```python
from build123d import *

# Parameters (mm, degrees)
SKETCH_1_R               = 3.5
SKETCH_1_R_2             = 2.5
EXTRUDE_1_DEPTH          = 3
CHAMFER_1_SIZE           = 0.1
CUT_EXTRUDE_2_DEPTH      = 6.787918451
CUT_EXTRUDE_2_DEPTH_BACK = 6.787918451
SKETCH_2_W               = 1
SKETCH_2_H               = 3.5


with BuildPart() as part:
    # 草图1 → 拉伸-薄壁1 (new body)
    with BuildSketch(Plane.XY):
        Circle(SKETCH_1_R)
        Circle(SKETCH_1_R_2, mode=Mode.SUBTRACT)
    extrude(amount=EXTRUDE_1_DEPTH)

    # 倒角1
    chamfer_1_edges = [part.edges().sort_by_distance(p)[0] for p in [
        (-3.5, 0, 0),
        (-2.5, 0, 0),
        (-3.5, 0, 3),
        (-2.5, 0, 3),
    ]]
    chamfer(chamfer_1_edges, length=CHAMFER_1_SIZE)

    # 草图2 → 切除-拉伸-薄壁2 (cut, two sides: drawn at the far end of the back side and taken through both)
    with BuildSketch(Plane(origin=(0, 0, 0), x_dir=(-1, 0, 0), z_dir=(0, 0, -1)).offset(-CUT_EXTRUDE_2_DEPTH_BACK)):
        with Locations((0, 1.75)):
            Rectangle(SKETCH_2_W, SKETCH_2_H)
    extrude(amount=CUT_EXTRUDE_2_DEPTH + CUT_EXTRUDE_2_DEPTH_BACK, mode=Mode.SUBTRACT)


solid = part.part
```
Build history of the part. All positions in model axes, mm. A direction names the side the tool comes from. Round coordinates to 2 decimals unless told otherwise and drop trailing zeros. Order: outer loops, then holes, each group sorted by start corner. A loop starts at its lowest first (then second) coordinate and runs counter-clockwise, first axis right, second up. Notation, with made-up numbers: (-39, -22.5) -> (-27, -22.5) arc R19 cw to (-27, -18.5) -> close; hole circle Ø9 at (0.25, -21). An arc over 180 degrees is marked (long way). Answer in a Markdown table with one row per item.
1) Band-saw the part on A-A on y = 0. Give the cut face in (x, z), and give its area (3 significant figures).
Values:
| item | result |
|---|---|
| outline | (-3.5, 0.1) -> (-3.4, 0) -> (-2.6, 0) -> (-2.5, 0.1) -> (-2.5, 2.9) -> (-2.6, 3) -> (-3.4, 3) -> (-3.5, 2.9) -> close; (2.5, 0.1) -> (2.6, 0) -> (3.4, 0) -> (3.5, 0.1) -> (3.5, 2.9) -> (3.4, 3) -> (2.6, 3) -> (2.5, 2.9) -> close |
| area | 5.96 mm2 |
2) Band-saw the part on B-B on x = 0. Give the cut face in (y, z).
Values:
| item | result |
|---|---|
| outline | (-3.5, 0.1) -> (-3.4, 0) -> (-2.6, 0) -> (-2.5, 0.1) -> (-2.5, 2.9) -> (-2.6, 3) -> (-3.4, 3) -> (-3.5, 2.9) -> close |
3) Wall check: L1, parallel to X at y = 0, z = 1.9; L2, parallel to Y at x = 0, z = 2.15; L3, parallel to X at y = 3, z = 1. Give the ranges that are in metal, low to high.
Values:
| item | result |
|---|---|
| L1 | -3.5 to -2.5, 2.5 to 3.5 |
| L2 | -3.5 to -2.5 |
| L3 | -1.8 to -0.5, 0.5 to 1.8 |
4) Which spindle directions (+Z, -Z, +X, -X, +Y, -Y) get a long thin tool onto all of the face, cutting with end or side? Do faces 4 (the flat face through (0.5, 3, 2)), 5 (the flat face through (1, -3, 3)). Say none if no direction does.
Values:
| item | result |
|---|---|
| face 4 | +Z, -Z, +Y |
| face 5 | +Z, +X, -X, +Y, -Y |
5) Band-saw the part on C-C on z = 1.8. Give the cut face in (x, y), and give its area (3 significant figures).
Values:
| item | result |
|---|---|
| outline | (-0.5, 2.45) -> (-0.5, 3.46) arc R3.5 ccw (long way) to (0.5, 3.46) -> (0.5, 2.45) arc R2.5 cw (long way) to start |
| area | 17.8 mm2 |
6) Pin check, flat tips, straight feed: P1, Ø0.5, axis at y = 3, z = 1, coming from the +X side; P2, Ø1.5, axis at x = -1.5, z = 1.5, coming from the +Y side; P3, Ø1.5, axis at y = -0.5, z = 1.5, coming from the -X side; P4, Ø0.5, axis at y = 2.5, z = 1.5, coming from the -X side. Stop position of each tip, or through.
Values:
| item | result |
|---|---|
| P1 | x = 2.17 |
| P2 | y = 3.42 |
| P3 | x = -3.5 |
| P4 | x = -2.68 |
7) Mould opens along Y. For faces 1 (the cylindrical face through (-0.1, -2.5, 1.5)), 2 (the cylindrical face through (-0.1, -3.5, 1.5)), 3 (the flat face through (1, -3, 0)) say: released by +Y, released by -Y, zero draft, split by the parting line, or undercut.
Values:
| item | result |
|---|---|
| face 1 | undercut |
| face 2 | split by the parting line |
| face 3 | zero draft |
